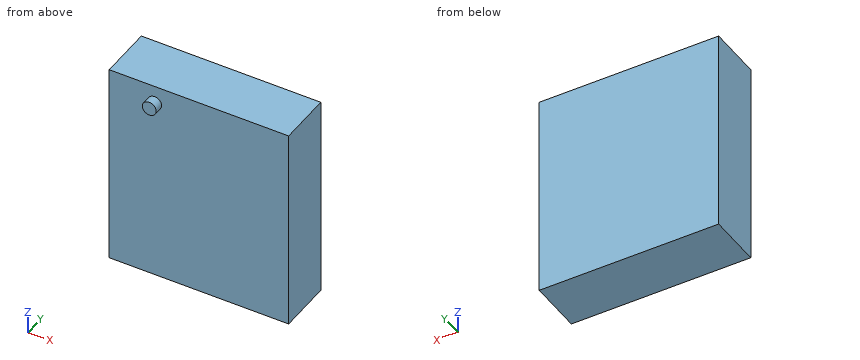
from build123d import *

# Parameters (mm, degrees)
SKETCH1_W           = 65.278
SKETCH1_H           = 75.184
BOSS_EXTRUDE1_DEPTH = 19.685
SKETCH3_R           = 2.54
BOSS_EXTRUDE2_DEPTH = 3.302


with BuildPart() as part:
    # Sketch1 → Boss-Extrude1 (new body)
    with BuildSketch(Plane(origin=(0, 0, 0), x_dir=(1, 0, 0), z_dir=(0, 1, 0))):
        with Locations((32.639, 37.592)):
            Rectangle(SKETCH1_W, SKETCH1_H)
    extrude(amount=BOSS_EXTRUDE1_DEPTH)

    # Sketch3 → Boss-Extrude2 (add)
    with BuildSketch(Plane.XZ):
        with Locations((16.51, -6.604)):
            Circle(SKETCH3_R)
    extrude(amount=BOSS_EXTRUDE2_DEPTH)


solid = part.part
Input: part model. Units: mm. Frame: model coordinates. Give positions to 0.01 mm unless a question says otherwise; leave off trailing zeros. Write each loop counter-clockwise with the first axis right and the second up, starting at its lowest first coordinate (ties: lowest second). Pieces come first, ordered by that corner, then holes. Notation, with made-up numbers: M 72,43.5 L 97,43.5 A10 ccw 97,51.5 Z; hole C -2,35.5 d1. An arc over 180 degrees is marked long. Write item = value, one per line. Start each with the question number.
1) Material intervals for line 1 along Y through (x, z) = (5, -54.5) (3 decimals), sorted ascending. Write a range as [from, to].
2) Cut plane B-B on z = -63. Return the cut outline in (x, y) (3 decimals).
3) Cut plane C-C on y = -1.5. Return the cut outline in (x, z).
4) Cut plane A-A on x = 16.51. Return the cut outline in (y, z) (3 decimals).
5) First-contact query: pin 1 Ø1 at (x, z) = (29.5, -63) entering from -Y. Flat tip, straight axial feed; report the tip coordinate or a pass-through.
6) Cut plane D-D on x = 56. Return the cut outline in (y, z) (3 decimals).
Solved:
q1.line_1 = [0, 19.685]
q2.outline = M 0,0 L 65.278,0 L 65.278,19.685 L 0,19.685 Z
q3.outline = C 16.51,-6.6 d5.08
q4.outline = M -3.302,-9.144 L 0,-9.144 L 0,-75.184 L 19.685,-75.184 L 19.685,0 L 0,0 L 0,-4.064 L -3.302,-4.064 Z
q5.pin_1 = 0
q6.outline = M 0,-75.184 L 19.685,-75.184 L 19.685,0 L 0,0 Z
